Geometry: final body of the model. Coordinates: model frame, mm. A direction names the side the tool comes from. Give positions to 0.01 mm unless a question says otherwise; leave off trailing zeros. Loops run counter-clockwise (first coordinate to the right, second up) from the corner with the lowest first, then second, coordinate; pieces in that order, holes last. Notation, with made-up numbers: (30, 12.5) - (68, 12.5) arc R10 cw to (68, 31.5) - close; hole circle Ø2 at (43, 20). An arc over 180 degrees is marked (long way). Use one line per item in the form item = value.
```python
from build123d import *

# Parameters (mm, degrees)
BOSS_EXTRUDE1_DEPTH      = 27
CUT_EXTRUDE1_DEPTH       = 29
CUT_EXTRUDE1_DEPTH_BACK  = 70
BOSS_EXTRUDE2_DEPTH      = 27
SKETCH9_W                = 14.166666667
SKETCH9_H                = 10
BOSS_EXTRUDE3_DEPTH      = 3
SKETCH10_W               = 30
SKETCH10_H               = 50
CUT_EXTRUDE7_DEPTH       = 326.898757285
SKETCH11_W               = 20
SKETCH11_H               = 50
CUT_EXTRUDE9_DEPTH       = 22
BOSS_EXTRUDE4_DEPTH      = 27
FILLET1_R                = 10
FILLET2_R                = 10
CUT_EXTRUDE10_DEPTH      = 367.89508037
CUT_EXTRUDE10_DEPTH_BACK = 367.89508037
SKETCH17_W               = 385
SKETCH17_H               = 2
SKETCH18_W               = 20
SKETCH18_H               = 50
CUT_EXTRUDE11_DEPTH      = 22
SHELL1_START             = 2
SHELL1_DEPTH             = 20
SHELL1_START_2           = -55
SHELL1_2_DEPTH           = 80
CUT_EXTRUDE12_DEPTH      = 335.559411764
CUT_EXTRUDE12_DEPTH_BACK = 335.559411764
SKETCH20_W               = 70
SKETCH20_H               = 17


with BuildPart() as part:
    # Sketch1 → Boss-Extrude1 (new body)
    with BuildSketch(Plane(origin=(0, 0, 0), x_dir=(1, 0, 0), z_dir=(0, 1, 0))):
        Polygon((-30, 0), (-55, -30), (-15, -30), (-15, 0), align=None)
        Polygon((-15, 0), (-15, -30), (25, -30), (0, 0), align=None)
    extrude(amount=BOSS_EXTRUDE1_DEPTH)

    # Sketch3 → Cut-Extrude1 (cut, two sides: drawn at the far end of the back side and taken through both)
    with BuildSketch(Plane(origin=(0, 0, 0), x_dir=(0, 0, -1), z_dir=(1, 0, 0)).offset(-CUT_EXTRUDE1_DEPTH_BACK)):
        Polygon((-30, 0), (0, 27), (-30, 27), align=None)
    extrude(amount=CUT_EXTRUDE1_DEPTH + CUT_EXTRUDE1_DEPTH_BACK, mode=Mode.SUBTRACT)

    # Sketch5 → Boss-Extrude2 (add)
    with BuildSketch(Plane(origin=(0, 0, 0), x_dir=(1, 0, 0), z_dir=(0, 1, 0))):
        Polygon((-55, -30), (-75, -54), (-75, 316), (45, 316), (45, -54), (25, -30), (0, 0), (-30, 0), align=None)
    extrude(amount=BOSS_EXTRUDE2_DEPTH)

    # Sketch9 → Boss-Extrude3 (add)
    with BuildSketch(Plane(origin=(0, 27, 0), x_dir=(1, 0, 0), z_dir=(0, 1, 0))):
        with Locations((-67.916666667, -32)):
            Rectangle(SKETCH9_W, SKETCH9_H)
    extrude(amount=BOSS_EXTRUDE3_DEPTH)

    # Sketch10 → Cut-Extrude7 (cut, through all)
    with BuildSketch(Plane(origin=(0, 27, 0), x_dir=(1, 0, 0), z_dir=(0, 1, 0))):
        with Locations((-15, 25)):
            Rectangle(SKETCH10_W, SKETCH10_H)
    extrude(amount=-CUT_EXTRUDE7_DEPTH, mode=Mode.SUBTRACT)

    # Sketch11 → Cut-Extrude9 (cut)
    with BuildSketch(Plane(origin=(0, 27, 0), x_dir=(1, 0, 0), z_dir=(0, 1, 0))):
        with Locations((-40, 25)):
            Rectangle(SKETCH11_W, SKETCH11_H)
    extrude(amount=-CUT_EXTRUDE9_DEPTH, mode=Mode.SUBTRACT)

    # Sketch16 → Boss-Extrude4 (add)
    with BuildSketch(Plane(origin=(0, 27, 0), x_dir=(1, 0, 0), z_dir=(0, 1, 0))):
        Polygon((-75, -54), (-107, -69), (-107, -54), (-107, -44), (-75, -44), align=None)
    boss_extrude4 = extrude(amount=-BOSS_EXTRUDE4_DEPTH)

    # Mirror1: Boss-Extrude4 across plane
    add(boss_extrude4.mirror(Plane.ZY.offset(15)))

    # Fillet1
    fillet1_edges = [part.edges().sort_by_distance(p)[0] for p in [
        (-75, 13.5, 54),
    ]]
    fillet(fillet1_edges, radius=FILLET1_R)

    # Fillet2
    fillet2_edges = [part.edges().sort_by_distance(p)[0] for p in [
        (45, 13.5, 54),
    ]]
    fillet(fillet2_edges, radius=FILLET2_R)

    # Sketch17 → Cut-Extrude10 (cut, two sides: drawn at the far end of the back side and taken through both)
    with BuildSketch(Plane(origin=(77, 0, 0), x_dir=(0, 0, -1), z_dir=(1, 0, 0)).offset(-CUT_EXTRUDE10_DEPTH_BACK)):
        with Locations((123.5, 1)):
            Rectangle(SKETCH17_W, SKETCH17_H)
    extrude(amount=CUT_EXTRUDE10_DEPTH + CUT_EXTRUDE10_DEPTH_BACK, mode=Mode.SUBTRACT)

    # Sketch18 → Cut-Extrude11 (cut)
    with BuildSketch(Plane(origin=(0, 27, 0), x_dir=(1, 0, 0), z_dir=(0, 1, 0))):
        with Locations((10, 25)):
            Rectangle(SKETCH18_W, SKETCH18_H)
    extrude(amount=-CUT_EXTRUDE11_DEPTH, mode=Mode.SUBTRACT)

    # Shell1: read off the stored shape, not the designer's step
    # Shell1 outline → Shell1 (cut)
    with BuildSketch(Plane(origin=(0, 0, 0), x_dir=(1, 0, 0), z_dir=(0, 1, 0)).offset(SHELL1_START)):
        Polygon((25, 55), (25, -5), (10.675208063, -5), (40, -40.189750324), (40, 311), (-70, 311), (-70, -40.189750324), (-40.675208063, -5), (-55, -5), (-55, 55), align=None)
        with BuildLine():
            Line((47.34187473, -49), (47.417185838, -49.090373329))
            ThreePointArc((47.417185838, -49.090373329), (48.203790537, -49.847988861), (49.136122855, -50.416746011))
            Line((49.136122855, -50.416746011), (72, -61.134188423))
            Line((72, -61.134188423), (72, -49))
            Line((72, -49), (47.34187473, -49))
        make_face()
        with BuildLine():
            Line((-77.417185838, -49.090373329), (-77.34187473, -49))
            Line((-77.34187473, -49), (-102, -49))
            Line((-102, -49), (-102, -61.134188423))
            Line((-102, -61.134188423), (-79.136122855, -50.416746011))
            ThreePointArc((-79.136122855, -50.416746011), (-78.203790537, -49.847988861), (-77.417185838, -49.090373329))
        make_face()
    extrude(amount=SHELL1_DEPTH, mode=Mode.SUBTRACT)

    # Shell1 2 outline → Shell1 2 (cut)
    with BuildSketch(Plane.YZ.offset(SHELL1_START_2)):
        Polygon((2, 5), (15.773187976, 5), (2, 20.303542196), align=None)
    extrude(amount=SHELL1_2_DEPTH, mode=Mode.SUBTRACT)

    # Sketch20 → Cut-Extrude12 (cut, two sides: drawn at the far end of the back side and taken through both)
    with BuildSketch(Plane(origin=(0, 27, 0), x_dir=(1, 0, 0), z_dir=(0, 1, 0)).offset(-CUT_EXTRUDE12_DEPTH_BACK)):
        with Locations((-15, 58.5)):
            Rectangle(SKETCH20_W, SKETCH20_H)
    extrude(amount=CUT_EXTRUDE12_DEPTH + CUT_EXTRUDE12_DEPTH_BACK, mode=Mode.SUBTRACT)


solid = part.part
```
(1) Access query for faces 1 (the face through (-75, 16, -133)), 2 (the face through (10, 5, -25)), 3 (the face through (-91.797, 14.675, 61.874)), 4 (the face through (-89, 27, 53)), 5 (the face through (-14, 12, -311)). Directions: +Z, -Z, +X, -X, +Y, -Y. A direction counts if a zero-diameter tool reaches every point of the face in a straight line with its end or side. Return the directions, or none.
Solution:
face_1 = -Z, -X, +Y, -Y
face_2 = +Y
face_3 = +Z, +Y, -Y
face_4 = +Z, +X, -X, +Y
face_5 = -Y
(2) Cut plane A-A (x = -3.5). Return the cut outline in (y, z), plus the area to 3 significant figures.
Solution:
outline = (2, -316) - (27, -316) - (27, -67) - (22, -67) - (22, -311) - (2, -311) - close; (2, 0) - (27, 0) - (2, 27.78) - (2, 20.3) - (15.77, 5) - (2, 5) - close
area = 1,590 mm2
(3) Pin query (flat end, axial travel): P1, Ø1, axis at x = -76, y = 8.5, coming from the +Z side; P2, Ø5, axis at x = -31.5, y = 15.5, coming from the +Z side; P3, Ø6, axis at x = -10.5, y = 17, coming from the +Z side. Return the tip coordinate at first contact, or that it passes through.
Solution:
P1 = 54.68
P2 = 15.56
P3 = 14.44
(4) Cut plane C-C (y = 9.25). Give the number of separate pieces and of enclosed holes in the cut face, plus the area to 3 significant figures.
Solution:
separate_pieces = 2
enclosed_holes = 3
area = 6,810 mm2
(5) Cut plane B-B (z = -181). Return the cut outline in (x, y), plus the area to 3 significant figures.
Solution:
outline = (-75, 2) - (-70, 2) - (-70, 22) - (40, 22) - (40, 2) - (45, 2) - (45, 27) - (-75, 27) - close
area = 800 mm2
(6) Pull-direction query (Z, two-part tool) for faces 6 (the face through (61.797, 14.675, 61.874)), 7 (the face through (-33, 2, -18)), 8 (the face through (-15.538, 8.983, 12.545)); classes: released by +Z, released by -Z, zero draft, split by the parting line, or undercut.
Solution:
face_6 = released by +Z
face_7 = zero draft
face_8 = undercut
(7) Material intervals for L1, parallel to X at y = 17.5, z = -50; L2, parallel to X at y = 5.25, z = -276; L3, parallel to Z at x = -46.5, y = 21.25, sorted ascending. Write a range as from..to.
Solution:
L1 = -75..-70, -55..-50, 20..25, 40..45
L2 = -75..-70, 40..45
L3 = -316..-311, 0..5, 11.99..19.8
(8) Cut plane D-D (x = 31). Return the cut outline in (y, z), plus the area to 3 significant figures.
Solution:
outline = (2, -316) - (27, -316) - (27, 37.2) - (2, 37.2) - (2, 29.39) - (22, 29.39) - (22, -311) - (2, -311) - close
area = 2,020 mm2
